Part model, mm, in its own coordinate system. A direction names the side the tool comes from. Give positions to 0.01 mm unless a question says otherwise; leave off trailing zeros. Order: outer loops, then holes, each group sorted by start corner. A loop starts at its lowest first (then second) coordinate and runs counter-clockwise, first axis right, second up. Notation, with made-up numbers: M -13.5,35.25 L 11.5,35.25 A23 ccw 11.5,52.25 Z; hole C 35.5,8 d2. An arc over 180 degrees is marked long. Write each question's results on one line, items separated by ' | '. Start each with the question number.
from build123d import *

# Parameters (mm, degrees)
SKETCH_R  = 1
PAD_DEPTH = 3


with BuildPart() as part:
    # Sketch → Pad (new body)
    with BuildSketch(Plane.XY):
        Polygon((0, 0), (8, 0), (10, 3), (16, 3), (18, 0), (26, 0), (28, 3), (28, 5), (30, 5), (30, 6.5), (-3, 21), (-8, 21), (-8, 5), (-2, 5), (-2, 3), align=None)
        with Locations((-5, 19)):
            Circle(SKETCH_R, mode=Mode.SUBTRACT)
        with Locations((-5, 15.5)):
            Circle(SKETCH_R, mode=Mode.SUBTRACT)
        with Locations((-5, 12)):
            Circle(SKETCH_R, mode=Mode.SUBTRACT)
    extrude(amount=PAD_DEPTH)


solid = part.part
(1) Probe L1, parallel to Y at x = -5, z = 0.75; L2, parallel to X at y = 1.25, z = 2.1; L3, parallel to Y at x = 13, z = 1.25. List the from-to ranges inside material, lowest first.
(2) Pull direction Y, two halves, no side cores. Call faces 1 (the cylindrical face through (-5.217, 14.524, 1.479)), 2 (the flat face through (-2, 4, 1)), 3 (the flat face through (17, 1.5, 1.5)): +Y half, -Y half, draft (parallel to the pull), parting line (faces both ways), or undercut.
(3) Saw through at D-D on y = 12. Give the cut face in (x, z).
(4) Drop flat-ended pins along their axis: P1, Ø0.6, axis at x = 29.5, z = 2, coming from the -Y side; P2, Ø2.5, axis at x = -5, y = 15.5, coming from the +Z side; P3, Ø0.6, axis at y = 3.5, z = 1, coming from the +X side. Give the stop position or say it passes through.
(5) Saw through at C-C on x = -5. Give the cut face in (y, z).
(6) Tool access for faces 4 (the flat face through (-8, 13, 1)), 5 (the flat face through (29, 5, 1)), 6 (the flat face through (-5, 5, 1)), 7 (the flat face through (9, 1.5, 1.5)): list every direction of +Z, -Z, +X, -X, +Y, -Y with a clear straight run to the whole face (end or side of a thin tool).
(7) Saw through at A-A on z = 0.8. Give the cut face in (x, y), plus the area to 3 significant figures.
(8) Saw through at B-B on y = 18.5. Give the cut face in (x, z).
Taken from the geometry:
1) L1: y = 5 to 11, 13 to 14.5, 16.5 to 18, 20 to 21 | L2: x = -0.83 to 8.83, 17.17 to 26.83 | L3: y = 3 to 13.97
2) face 1: undercut | face 2: draft | face 3: -Y half
3) outline: M -8,0 L -6,0 L -6,3 L -8,3 Z; M -4,0 L 17.48,0 L 17.48,3 L -4,3 Z
4) P1: stops at y = 5 | P2: stops at z = 3 | P3: stops at x = 28
5) outline: M 5,0 L 11,0 L 11,3 L 5,3 Z; M 13,0 L 14.5,0 L 14.5,3 L 13,3 Z; M 16.5,0 L 18,0 L 18,3 L 16.5,3 Z; M 20,0 L 21,0 L 21,3 L 20,3 Z
6) face 4: +Z, -Z, -X, +Y, -Y | face 5: +Z, -Z, +X, -Y | face 6: +Z, -Z, -X, -Y | face 7: +Z, -Z, -Y
7) outline: M -8,5 L -2,5 L -2,3 L 0,0 L 8,0 L 10,3 L 16,3 L 18,0 L 26,0 L 28,3 L 28,5 L 30,5 L 30,6.5 L -3,21 L -8,21 Z; hole C -5,12 d2; hole C -5,15.5 d2; hole C -5,19 d2 | area: 479 mm²
8) outline: M -8,0 L -5.87,0 L -5.87,3 L -8,3 Z; M -4.13,0 L 2.69,0 L 2.69,3 L -4.13,3 Z
